Geometry check sheet. Reference: the model listing, model coordinates, mm. Face numbers are marked on the shaded views. A direction names the side the tool comes from. Give positions to 0.01 mm unless a question says otherwise; leave off trailing zeros. Write each loop counter-clockwise with the first axis right and the second up, starting at its lowest first coordinate (ties: lowest second). Pieces come first, ordered by that corner, then holes. Notation, with made-up numbers: (24.25, -16) -> (42.25, -16) arc R23 cw to (42.25, 2) -> close; hole circle Ø3 at (65, 49). An arc over 180 degrees is marked (long way). Use a Markdown table: item, result. Add a question column.
from build123d import *

# Parameters (mm, degrees)
SKETCH_W        = 100
SKETCH_H        = 70
PAD_DEPTH       = 3
SKETCH001_W     = 100
SKETCH001_H     = 3
PAD001_DEPTH    = 50
SKETCH002_W     = 3
SKETCH002_H     = 70
PAD002_DEPTH    = 50
POCKET_DEPTH    = 4
SKETCH004_R     = 2.5
POCKET001_DEPTH = 4
SKETCH005_W     = 12.7
SKETCH005_H     = 9
POCKET002_DEPTH = 4


with BuildPart() as part:
    # Sketch → Pad (new body)
    with BuildSketch(Plane.XY):
        with Locations((50, 35)):
            Rectangle(SKETCH_W, SKETCH_H)
    extrude(amount=PAD_DEPTH)

    # Sketch001 (on Face6 of Pad) → Pad001 (join)
    with BuildSketch(Plane.XY.offset(3)):
        with Locations((50, 68.5)):
            Rectangle(SKETCH001_W, SKETCH001_H)
        with Locations((50, 1.5)):
            Rectangle(SKETCH001_W, SKETCH001_H)
    extrude(amount=PAD001_DEPTH)

    # Sketch002 (on Face8 of Pad001) → Pad002 (join)
    with BuildSketch(Plane.XY.offset(3)):
        with Locations((1.5, 35)):
            Rectangle(SKETCH002_W, SKETCH002_H)
        with Locations((98.5, 35)):
            Rectangle(SKETCH002_W, SKETCH002_H)
    extrude(amount=PAD002_DEPTH)

    # Sketch003 (on Face6 of Pad002) → Pocket (cut)
    with BuildSketch(Plane(origin=(0, 70, 0), x_dir=(-1, 0, 0), z_dir=(0, 1, 0))):
        with BuildLine():
            ThreePointArc((-71.997929, 31.001554), (-75, 40), (-78.002071, 31.001554))
            Line((-78.002071, 31.001554), (-71.997929, 31.001554))
        make_face()
        with BuildLine():
            ThreePointArc((-21.937304, 31.047799), (-25, 40), (-28.062696, 31.047799))
            Line((-28.062696, 31.047799), (-21.937304, 31.047799))
        make_face()
    extrude(amount=-POCKET_DEPTH, mode=Mode.SUBTRACT)

    # Sketch004 (on Face23 of Pocket) → Pocket001 (cut)
    with BuildSketch(Plane.XZ):
        with Locations((17.5, 25)):
            Circle(SKETCH004_R)
        with Locations((32.5, 25)):
            Circle(SKETCH004_R)
        with Locations((67.5, 25)):
            Circle(SKETCH004_R)
        with Locations((82.5, 25)):
            Circle(SKETCH004_R)
    extrude(amount=-POCKET001_DEPTH, mode=Mode.SUBTRACT)

    # Sketch005 (on Face6 of Pocket001) → Pocket002 (cut)
    with BuildSketch(Plane(origin=(0, 70, 0), x_dir=(-1, 0, 0), z_dir=(0, 1, 0))):
        with Locations((-83.65, 12.5)):
            Rectangle(SKETCH005_W, SKETCH005_H)
    extrude(amount=-POCKET002_DEPTH, mode=Mode.SUBTRACT)


solid = part.part
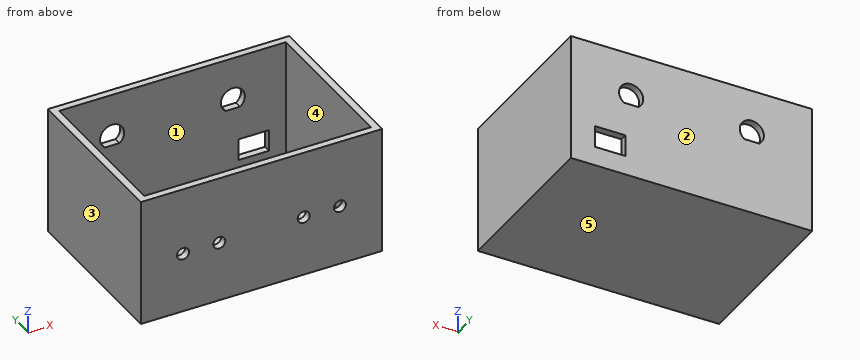
1) Sectioned sample at C-C, the plane y = 37.5. Enter the section's corners in (x, z).
2) Sectioned sample at A-A, the plane z = 21. Enter the section's corners in (x, y), and give its area (3 significant figures).
3) Sectioned sample at B-B, the plane x = 82.5. Enter the section's corners in (y, z), and give its area (3 significant figures).
4) Draft check along X on the marked faces 1, 2 and 3. Enter one of: +X half, -X half, draft (parallel to the pull), parting line (faces both ways), or undercut.
5) Material ranges on probe 1 along X at (y, z) = (68, 35); probe 2 along X at (y, z) = (46.5, 37.5); probe 3 along Y at (x, z) = (32.5, 6.5), recorded low to high. Write a range as [from, to].
6) Gauge pin test, flat ends, axial feed: P1, Ø4, axis at x = 67.5, z = 25, coming from the -Y side; P2, Ø5, axis at x = 75, y = 14, coming from the +Z side. Record the tip position at first contact, or that the pin passes through.
7) Tool access check on the marked faces 4 and 5. Record the directions out of +Z, -Z, +X, -X, +Y, -Y that give a thin tool (end or side, any length) a straight path to the whole face; none if there is none.
8) Sectioned sample at D-D, the plane x = 25. Enter the section's corners in (y, z), and give its area (3 significant figures).
Check values:
| question | item | result |
|---|---|---|
| 1 | outline | (0, 0) -> (100, 0) -> (100, 53) -> (97, 53) -> (97, 3) -> (3, 3) -> (3, 53) -> (0, 53) -> close |
| 2 | outline | (0, 0) -> (100, 0) -> (100, 70) -> (0, 70) -> close; hole (3, 3) -> (97, 3) -> (97, 67) -> (3, 67) -> close |
| 2 | area | 984 mm² |
| 3 | outline | (0, 0) -> (70, 0) -> (70, 8) -> (67, 8) -> (67, 3) -> (3, 3) -> (3, 22.5) -> (0, 22.5) -> close; (0, 27.5) -> (3, 27.5) -> (3, 53) -> (0, 53) -> close; (67, 17) -> (70, 17) -> (70, 53) -> (67, 53) -> close |
| 3 | area | 468 mm² |
| 4 | face 1 | undercut |
| 4 | face 2 | draft |
| 4 | face 3 | -X half |
| 5 | probe 1 | [0, 20], [30, 70], [80, 100] |
| 5 | probe 2 | [0, 3], [97, 100] |
| 5 | probe 3 | [0, 3], [67, 70] |
| 6 | P1 | y = 67 |
| 6 | P2 | z = 3 |
| 7 | face 4 | +Z |
| 7 | face 5 | -Z, +X, -X, +Y, -Y |
| 8 | outline | (0, 0) -> (70, 0) -> (70, 31.05) -> (67, 31.05) -> (67, 3) -> (3, 3) -> (3, 53) -> (0, 53) -> close; (67, 40) -> (70, 40) -> (70, 53) -> (67, 53) -> close |
| 8 | area | 483 mm² |
